from build123d import *

# Parameters (mm, degrees)
SKETCH1_R           = 2.5
BOSS_EXTRUDE1_DEPTH = 3


with BuildPart() as part:
    # Sketch1 → Boss-Extrude1 (new body)
    with BuildSketch(Plane.XY):
        with BuildLine():
            Line((0, 10), (10, 10))
            ThreePointArc((10, 10), (12.121320344, 9.121320344), (13, 7))
            Line((13, 7), (13, 3))
            ThreePointArc((13, 3), (12.121320344, 0.878679656), (10, 0))
            Line((10, 0), (0, 0))
            Line((0, 0), (0, 3))
            Line((0, 3), (3, 3))
            Line((3, 3), (3, 7))
            Line((3, 7), (0, 7))
            Line((0, 7), (0, 10))
        make_face()
        with Locations((8, 5)):
            Circle(SKETCH1_R, mode=Mode.SUBTRACT)
    extrude(amount=BOSS_EXTRUDE1_DEPTH)


solid = part.part
Input: part model. Units: mm. Frame: model coordinates. A direction names the side the tool comes from. Round coordinates to 2 decimals unless told otherwise and drop trailing zeros. Order: outer loops, then holes, each group sorted by start corner. A loop starts at its lowest first (then second) coordinate and runs counter-clockwise, first axis right, second up. Notation, with made-up numbers: (-3, 31.25) - (36, 31.25) arc R23 ccw to (36, 42.25) - close; hole circle Ø2 at (21.25, -24). An arc over 180 degrees is marked (long way). Use a Markdown table: item, result.
1. Section B-B on z = 2.25. Return the cut outline in (x, y).
Evaluation:
| item | result |
|---|---|
| outline | (0, 0) - (10, 0) arc R3 ccw to (13, 3) - (13, 7) arc R3 ccw to (10, 10) - (0, 10) - (0, 7) - (3, 7) - (3, 3) - (0, 3) - close; hole circle Ø5 at (8, 5) |
2. Mould query, pull axis Y, two halves, no side actions, for faces 1 (the face through (2, 7, 1)), 2 (the face through (5, 0, 1)), 3 (the face through (12.1, 9.14, 1.48)). Classes: +Y half, -Y half, draft (parallel to the pull), parting line (faces both ways), or undercut.
Evaluation:
| item | result |
|---|---|
| face 1 | undercut |
| face 2 | -Y half |
| face 3 | +Y half |
3. Access query for faces 4 (the face through (5, 5, 3)), 5 (the face through (1, 3, 1)). Directions: +Z, -Z, +X, -X, +Y, -Y. A direction counts if a zero-diameter tool reaches every point of the face in a straight line with its end or side. Return the directions, or none.
Evaluation:
| item | result |
|---|---|
| face 4 | +Z, +X, -X, +Y, -Y |
| face 5 | +Z, -Z, -X |
4. Section C-C on y = 6.25. Return the cut outline in (x, z).
Evaluation:
| item | result |
|---|---|
| outline | (3, 0) - (5.83, 0) - (5.83, 3) - (3, 3) - close; (10.17, 0) - (13, 0) - (13, 3) - (10.17, 3) - close |
5. Material intervals for probe 1 along Y at (x, z) = (8, 1.6); probe 2 along Y at (x, z) = (6.5, 0.9); probe 3 along X at (y, z) = (6, 2.75), sorted ascending.
Evaluation:
| item | result |
|---|---|
| probe 1 | 0 to 2.5, 7.5 to 10 |
| probe 2 | 0 to 3, 7 to 10 |
| probe 3 | 3 to 5.71, 10.29 to 13 |
6. Section A-A on x = 8. Return the cut outline in (y, z).
Evaluation:
| item | result |
|---|---|
| outline | (0, 0) - (2.5, 0) - (2.5, 3) - (0, 3) - close; (7.5, 0) - (10, 0) - (10, 3) - (7.5, 3) - close |
7. Section D-D on y = 9. Return the cut outline in (x, z).
Evaluation:
| item | result |
|---|---|
| outline | (0, 0) - (12.24, 0) - (12.24, 3) - (0, 3) - close |
